```python
from build123d import *

# Parameters (mm, degrees)
F1_DEPTH        = 18
F2_R            = 18.5
F4_DEPTH        = 34.5
F5_R            = 15
F7_DEPTH        = 34.5
F11_D           = 11
F11_CBORE_D     = 17.25
F11_CBORE_DEPTH = 10
F14_D           = 11
F14_CBORE_D     = 17.25
F14_CBORE_DEPTH = 10
F15_R           = 2


with BuildPart() as f1:
    # F0 (on Front) → F1 (new body, symmetric)
    with BuildSketch(Plane.XZ):
        Polygon((-88.5, 0), (0, 0), (0, 26.5), (-51.5, 26.5), (-51.5, 36.5), (-88.5, 36.5), align=None)
    extrude(amount=F1_DEPTH, both=True)

    # F2
    f2_edges = [f1.edges().sort_by_distance(p)[0] for p in [
        (0, 0, 26.5),
        (-88.5, 0, 0),
    ]]
    fillet(f2_edges, radius=F2_R)

    # F3 (on face) → F4 (join)
    with BuildSketch(Plane.YZ):
        with BuildLine():
            Line((-41.0676798294, -22.9138953121), (-33.4179196431, -36.1636686207))
            ThreePointArc((-33.4179196431, -36.1636686207), (0, -23), (33.4179196431, -36.1636686207))
            Line((33.4179196431, -36.1636686207), (41.0676798294, -22.9138953121))
            ThreePointArc((41.0676798294, -22.9138953121), (30.1704829466, -15.557622669), (18, -10.5833898689))
            ThreePointArc((18, -10.5833898689), (0, -8), (-18, -10.5833898689))
            ThreePointArc((-18, -10.5833898689), (-30.1704829466, -15.557622669), (-41.0676798294, -22.9138953121))
        make_face()
        with BuildLine():
            Line((-18, 0), (-18, -10.5833898689))
            ThreePointArc((-18, -10.5833898689), (0, -8), (18, -10.5833898689))
            Line((18, -10.5833898689), (18, 0))
            Line((18, 0), (-18, 0))
        make_face()
    extrude(amount=-F4_DEPTH)

    # F5
    f5_edges = [f1.edges().sort_by_distance(p)[0] for p in [
        (-17.25, -18, -10.58339),
        (-17.25, 18, -10.58339),
    ]]
    fillet(f5_edges, radius=F5_R)

    # F6 (on face) → F7 (join)
    with BuildSketch(Plane.YZ):
        Polygon((-41.0676798294, -22.9138953121), (-26.7341772152, -13.8511928873), (-42.1958866534, -20.9597837716), align=None)
        Polygon((42.1958866534, -20.9597837716), (26.7341772152, -13.8511928873), (41.0676798294, -22.9138953121), align=None)
    extrude(amount=-F7_DEPTH)

    # F11 (through all)
    with Locations(Plane(origin=(0, -0.1973911234, 0.4293402511), x_dir=(1, 0, 0), z_dir=(0, -0.417721519, 0.9085751111))):
        with Locations((-17.25, -33.8857312325)):
            CounterBoreHole(F11_D / 2, F11_CBORE_D / 2, F11_CBORE_DEPTH)

    # F14 (through all)
    with Locations(Plane(origin=(0, 0.1973911234, 0.4293402511), x_dir=(1, 0, 0), z_dir=(0, 0.417721519, 0.9085751111))):
        with Locations((-17.25, 33.8857312325)):
            CounterBoreHole(F14_D / 2, F14_CBORE_D / 2, F14_CBORE_DEPTH)

    # F15
    f15_edges = [f1.edges().sort_by_distance(p)[0] for p in [
        (0, -37.806903, -28.561726),
        (-17.25, -42.195887, -20.959784),
        (-34.5, -37.806903, -28.561726),
        (-17.25, 42.195887, -20.959784),
        (0, 37.806903, -28.561726),
        (-34.5, 37.806903, -28.561726),
    ]]
    fillet(f15_edges, radius=F15_R)


solid = f1.part
```
Check sheet for the modelled part. Datum: model origin and axes. Units: mm. A direction names the side the tool comes from. Round coordinates to 2 decimals unless told otherwise and drop trailing zeros. Loops run counter-clockwise (first coordinate to the right, second up) from the corner with the lowest first, then second, coordinate; pieces in that order, holes last. Notation, with made-up numbers: (-24, 86) - (-8, 86) arc R10 cw to (-8, 103) - close; hole circle Ø5 at (42.25, 63.5). An arc over 180 degrees is marked (long way). Answer as a JSON object with one key per item and string values. Group by question number.
Q1. Mould release check, pull along X, two halves, no side actions. Record for faces 5 (the face through (-16.06, -30.04, -28.64)), 6 (the face through (-44, -18, 14)), 7 (the face through (0, -1, -13)): released by +X, released by -X, zero draft, split by the parting line, or undercut.
Q2. Sectioned sample at C-C, the plane z = -25. Count the separate pieces of the cut face and the enclosed holes in it, plus the area to 3 significant figures.
Q3. Scan lines: line 1 along X through (y, z) = (2, 30); line 2 along Y through (x, z) = (-49.5, 15); line 3 along X through (y, z) = (-6.5, -10). Record each from-to range of solid material in increasing order. Write a range as [from, to].
Q4. Sectioned sample at A-A, the plane x = -31. Enter the section's corners in (y, z).
Q5. Sectioned sample at D-D, the plane y = 7. Enter the section's corners in (x, z), plus the area to 3 significant figures.
Q6. Sectioned sample at B-B, the plane y = -12. Enter the section's corners in (x, z), plus the area to 3 significant figures.
Q7. Set-up check for faces 1 (the face through (-52, 0, 0)), 2 (the face through (-51.5, 0, 31)), 3 (the face through (-44, 18, 14)), 4 (the face through (-15.45, -31.92, -25.16)): record each of +Z, -Z, +X, -X, +Y, -Y from which the full face is reachable in a straight line by a thin tool's end or side.
Q8. Gauge pin test, flat ends, axial feed: P1, Ø10, axis at x = -40.5, z = 8, coming from the +Y side; P2, Ø8, axis at y = 23, z = -1.5, coming from the +X side; P3, Ø16.5, axis at x = -32.5, y = -2.5, coming from the +Z side; P4, Ø12, axis at x = -38.5, y = -21, coming from the -Z side. Record the tip position at first contact, or that the pin passes through.
Solution:
{
 "1": {"face 5": "undercut", "face 6": "zero draft", "face 7": "released by +X"},
 "2": {"separate pieces": "2", "enclosed holes": "2", "area": "1,510 mm²"},
 "3": {"line 1": "x = [-88.5, -51.5]", "line 2": "y = [-18, 18]", "line 3": "x = [-34.5, 0]"},
 "4": {"outline": "(-41.1, -22.86) - (-33.42, -36.16) arc R49 cw to (33.42, -36.16) - (41.1, -22.86) arc R2 ccw to (40.2, -20.04) - (26.73, -13.85) arc R15 cw to (18, -0.22) - (18, 26.5) - (-18, 26.5) - (-18, -0.22) arc R15 cw to (-26.73, -13.85) - (-40.2, -20.04) arc R2 ccw to start"},
 "5": {"outline": "(-88.5, 18.5) arc R18.5 ccw to (-70, 0) - (-34.5, 0) - (-34.5, -23.5) - (0, -23.5) - (0, 8) arc R18.5 ccw to (-18.5, 26.5) - (-51.5, 26.5) - (-51.5, 36.5) - (-88.5, 36.5) - close", "area": "3,380 mm²"},
 "6": {"outline": "(-88.5, 18.5) arc R18.5 ccw to (-70, 0) - (-34.5, 0) - (-34.5, -24.49) - (0, -24.49) - (0, 8) arc R18.5 ccw to (-18.5, 26.5) - (-51.5, 26.5) - (-51.5, 36.5) - (-88.5, 36.5) - close", "area": "3,410 mm²"},
 "7": {"face 1": "-Z, -X, +Y, -Y", "face 2": "+Z, +X, +Y, -Y", "face 3": "+Z, +X, -X, +Y", "face 4": "none"},
 "8": {"P1": "stops at y = 18", "P2": "passes through", "P3": "stops at z = 26.5", "P4": "stops at z = -30.14"}
}
